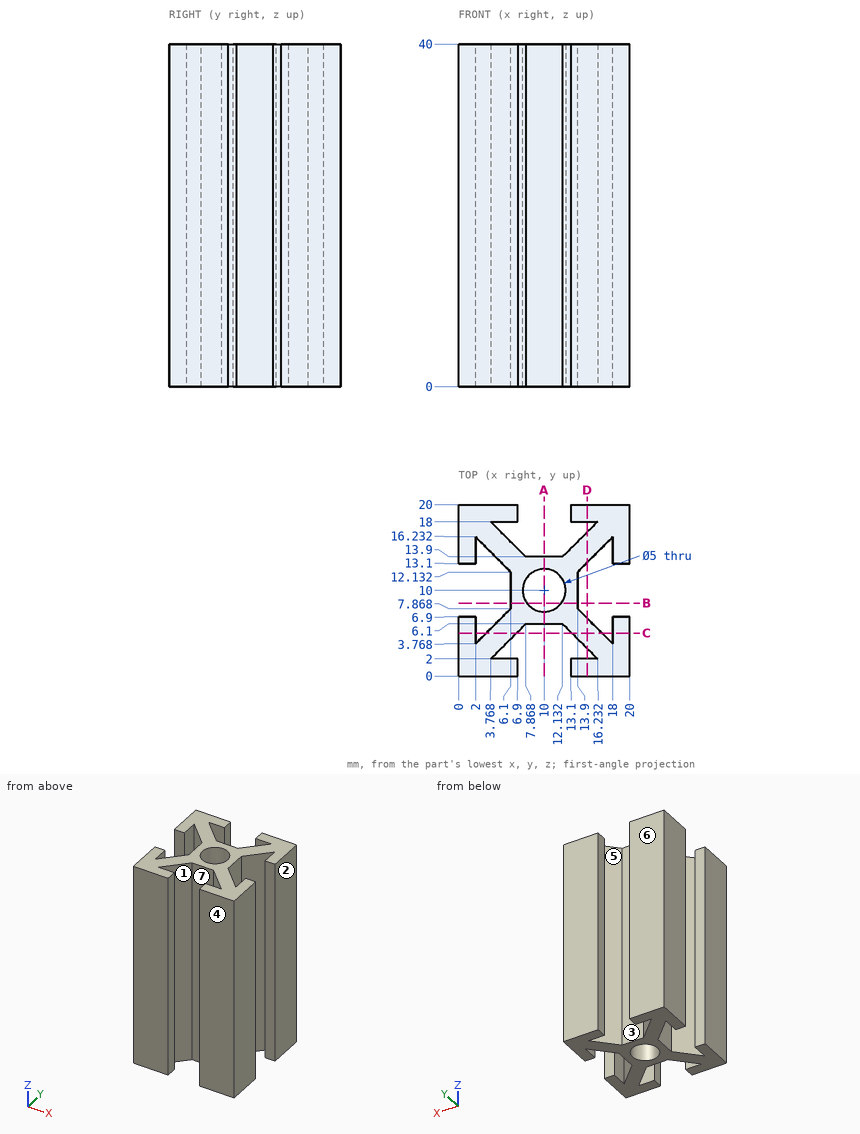
Here's the drawing with two shaded views (mm, measured from the low corner). I have some questions. A direction names the side the tool comes from. Coordinates: 2 decimals unless noted, no trailing zeros. Loops run counter-clockwise (first coordinate to the right, second up) from the corner with the lowest first, then second, coordinate; pieces in that order, holes last. Notation, with made-up numbers: (-19, 77.25) -> (-3, 77.25) arc R27 ccw to (-3, 94.25) -> close; hole circle Ø5 at (-31, -21). An arc over 180 degrees is marked (long way). Put each result on its own line as item: value. Start each with the question number.
Q1. If I drill on line 1 (Y direction, x = 10, z = 30); line 2 (Y direction, x = 16, z = 20.5); line 3 (X direction, y = 5.5, z = 33), over which ranges is the centre line in solid material (lowest first)? Write a range as [from, to].
Q2. I'm going to push flat-ended pins straight in: P1, Ø1.5, axis at y = 12, z = 16.5, coming from the -X side; P2, Ø2, axis at x = 10, z = 22.5, coming from the -Y side; P3, Ø1.3, axis at y = 9, z = 12.5, coming from the +X side. Where does each tip first touch, or does it pass through?
Q3. I want a section at B-B (y = 8.5). Write out the boundary of the cut face in (x, z), plus the area to 3 significant figures.
Q4. For the marked faces 5, 6 and 7, which set-ups out of +Z, -Z, +X, -X, +Y, -Y let a thin tool reach every point of the face, with its end or its side?
Q5. I want a section at A-A (x = 10). Write out the boundary of the cut face in (y, z), plus the area to 3 significant figures.
Q6. Thinking about a two-plate mould opening in Y: for the marked faces 1, 2, 3 and 4, which applies, pulls with the +Y half, pulls with the -Y half, needs draft (parallel to the pull), parting line crosses it, or undercut?
Q7. I want a section at C-C (y = 5). Write out the boundary of the cut face in (x, z).
Taken from the geometry:
1. line 1: y = [6.1, 7.5], [12.5, 13.9]
1. line 2: y = [0, 2], [2.23, 5.77], [14.23, 17.77], [18, 20]
1. line 3: x = [0, 2], [3.73, 7.27], [12.73, 16.27], [18, 20]
2. P1: stops at x = 5.48
2. P2: stops at y = 6.1
2. P3: stops at x = 13.9
3. outline: (6.1, 0) -> (8, 0) -> (8, 40) -> (6.1, 40) -> close; (12, 0) -> (13.9, 0) -> (13.9, 40) -> (12, 40) -> close
3. area: 152 mm2
4. face 5: +Z, -Z
4. face 6: +Z, -Z, +X, -X, +Y
4. face 7: +Z, -Z, -Y
5. outline: (6.1, 0) -> (7.5, 0) -> (7.5, 40) -> (6.1, 40) -> close; (12.5, 0) -> (13.9, 0) -> (13.9, 40) -> (12.5, 40) -> close
5. area: 112 mm2
6. face 1: undercut
6. face 2: needs draft
6. face 3: pulls with the +Y half
6. face 4: pulls with the -Y half
7. outline: (0, 0) -> (2, 0) -> (2, 40) -> (0, 40) -> close; (3.23, 0) -> (6.77, 0) -> (6.77, 40) -> (3.23, 40) -> close; (13.23, 0) -> (16.77, 0) -> (16.77, 40) -> (13.23, 40) -> close; (18, 0) -> (20, 0) -> (20, 40) -> (18, 40) -> close
